Geometry: final body of the model. Coordinates: model frame, mm. Coordinates: 2 decimals unless noted, no trailing zeros. Order: outer loops, then holes, each group sorted by start corner. A loop starts at its lowest first (then second) coordinate and runs counter-clockwise, first axis right, second up. Notation, with made-up numbers: M 44,80.5 L 88,80.5 A12 ccw 88,101.5 Z; hole C -35,8 d7. An arc over 180 degrees is marked long. Use CSV: the item, a comma, the result in double quotes. Start each with the question number.
Q1. Ray query, probe 1 along X at (y, z) = (-0.25, 2); probe 2 along Y at (x, z) = (-95.25, -0.5) (3 decimals); probe 3 along Y at (x, z) = (-95.25, 1.5) (3 decimals). Return the intervals inside material, ascending.
Q2. First-contact query: P1, Ø3, axis at x = -21, y = -2, coming from the +Z side; P2, Ø4.5, axis at x = -95.25, y = 0, coming from the -Z side (3 decimals); P3, Ø2, axis at x = -98, y = 0, coming from the +Z side (3 decimals). Flat tips, straight axial feed; report the tip coordinate or a pass-through.
Q3. Section query A-A, the plane x = -95.25. Output: boundary loops of the cut face in (y, z) (1 decimal).
Q4. Section query D-D, the plane x = -72. Output: boundary loops of the cut face in (y, z) (1 decimal), and give its area (3 significant figures).
Q5. Section query B-B, the plane y = 0. Output: boundary loops of the cut face in (x, z) (1 decimal).
Q6. Section query C-C, the plane z = -0.5. Output: boundary loops of the cut face in (x, y) (3 decimals), and give its area (3 significant figures).
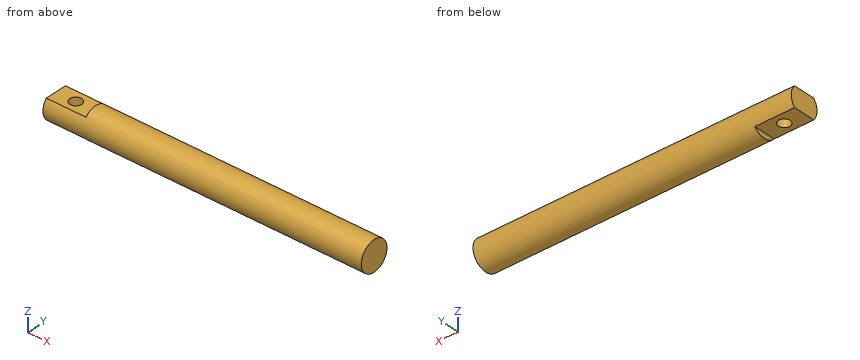
from build123d import *

# Parameters (mm, degrees)
SKETCH2_R               = 4.7625
BASE_EXTRUDE_DEPTH      = 101.6
CUT_EXTRUDE1_DEPTH      = 102.822997464
CUT_EXTRUDE1_DEPTH_BACK = 102.822997464
SKETCH5_R               = 1.905
CUT_EXTRUDE2_DEPTH      = 103.020808233


with BuildPart() as part:
    # Sketch2 → Base-Extrude (new body)
    with BuildSketch(Plane.ZY):
        Circle(SKETCH2_R)
    extrude(amount=BASE_EXTRUDE_DEPTH)

    # Sketch4 → Cut-Extrude1 (cut, two sides: drawn at the far end of the back side and taken through both)
    with BuildSketch(Plane(origin=(0, 0, 0), x_dir=(1, 0, 0), z_dir=(0, 1, 0)).offset(-CUT_EXTRUDE1_DEPTH_BACK)):
        Polygon((-109.22, 12.7), (-88.9, 12.7), (-88.9, 3.175), (-104.14, 3.175), (-104.14, -3.175), (-88.9, -3.175), (-88.9, -12.7), (-109.22, -12.7), align=None)
    extrude(amount=CUT_EXTRUDE1_DEPTH + CUT_EXTRUDE1_DEPTH_BACK, mode=Mode.SUBTRACT)

    # Sketch5 → Cut-Extrude2 (cut, through all)
    with BuildSketch(Plane.XY.offset(3.175)):
        with Locations((-95.25, 0)):
            Circle(SKETCH5_R)
    extrude(amount=-CUT_EXTRUDE2_DEPTH, mode=Mode.SUBTRACT)


solid = part.part
Responses:
1,probe 1,"x = -101.6 to -97.14, -93.36 to 0"
1,probe 2,"y = -4.736 to -1.905, 1.905 to 4.736"
1,probe 3,"y = -4.52 to -1.905, 1.905 to 4.52"
2,P1,"stops at z = 4.74"
2,P2,"stops at z = -3.175"
2,P3,"stops at z = 3.175"
3,outline,"M -3.5,-3.2 L -1.9,-3.2 L -1.9,3.2 L -3.5,3.2 A4.8 ccw Z; M 1.9,-3.2 L 3.5,-3.2 A4.8 ccw 3.5,3.2 L 1.9,3.2 Z"
4,outline,"C 0,0 d9.5"
4,area,"71.3 mm²"
5,outline,"M -101.6,-3.2 L -97.2,-3.2 L -97.2,3.2 L -101.6,3.2 Z; M -93.3,-3.2 L -88.9,-3.2 L -88.9,-4.8 L 0,-4.8 L 0,4.8 L -88.9,4.8 L -88.9,3.2 L -93.3,3.2 Z"
6,outline,"M -101.6,-4.736 L 0,-4.736 L 0,4.736 L -101.6,4.736 Z; hole C -95.25,0 d3.81"
6,area,"951 mm²"
